Build history of the part. All positions in model axes, mm. Give positions to 0.01 mm unless a question says otherwise; leave off trailing zeros. Loops run counter-clockwise (first coordinate to the right, second up) from the corner with the lowest first, then second, coordinate; pieces in that order, holes last.
1) Band-saw the part on B-B on y = 38.1. List the corners of the cut face in (x, z) (3 decimals).
2) Wall check: line 1 (Y direction, x = 1.25, z = 234) (3 decimals); line 2 (Y direction, x = 5.75, z = -272) (3 decimals); line 3 (Z direction, x = 1, y = 59). Give the ranges that are in metal, low to high.
3) Band-saw the part on A-A on z = -190. List the corners of the cut face in (x, y) (3 decimals).
4) Band-saw the part on C-C on x = 3. List the corners of the cut face in (y, z) (3 decimals), then the cut area to 3 significant figures.
Autodesk Inventor part; units mm, degrees
ref_plane "YZ Plane" through (0, 0, 0) normal (1, 0, 0) x (0, 1, 0)
ref_plane "XZ Plane" through (0, 0, 0) normal (0, 1, 0) x (-1, 0, 0)
ref_plane "XY Plane" through (0, 0, 0) normal (0, 0, 1) x (1, 0, 0)
sketch "Sketch1" plane through (0, 0, 0) normal (1, 0, 0) x (0, 1, 0)
  line L0 (-69.85, 342.9) -> (-69.85, -342.9)
  line L1 (-69.85, -342.9) -> (69.85, -342.9)
  line L2 (69.85, -342.9) -> (69.85, 342.9)
  line L3 (69.85, 342.9) -> (-69.85, 342.9)
  line L4 (-69.85, 342.9) -> (69.85, -342.9) construction
  line L5 (-69.85, -342.9) -> (69.85, 342.9) construction
  point P0 (0, 0)
  dimension "width" = 685.8
  dimension "height" = 139.7
extrude "Extrusion1" add sketch "Sketch1" along normal blind 6.35
sketch "Sketch2" plane through (6.35, 0, 0) normal (1, 0, 0) x (0, 0, -1)
  line L0 (-317.5, 38.1) -> (-63.5, 38.1) construction
  line L1 (-317.5, 28.575) -> (-63.5, 28.575)
  line L2 (-63.5, 47.625) -> (-317.5, 47.625)
  arc A0 (-317.5, 47.625) -> (-317.5, 28.575) centre (-317.5, 38.1) ccw
  arc A1 (-63.5, 28.575) -> (-63.5, 47.625) centre (-63.5, 38.1) ccw
  line L3 (342.9, 69.85) -> (-342.9, 69.85)
  line L4 (-342.9, 69.85) -> (-342.9, -69.85)
  line L5 (63.5, -38.1) -> (317.5, -38.1) construction
  line L6 (63.5, -47.625) -> (317.5, -47.625)
  line L7 (317.5, -28.575) -> (63.5, -28.575)
  arc A2 (63.5, -28.575) -> (63.5, -47.625) centre (63.5, -38.1) ccw
  arc A3 (317.5, -47.625) -> (317.5, -28.575) centre (317.5, -38.1) ccw
  line L8 (-342.9, -69.85) -> (342.9, -69.85)
  line L9 (342.9, -69.85) -> (342.9, 69.85)
  point P0 (0, 0)
  point P1 (-190.5, 38.1)
  point P2 (190.5, -38.1)
  dimension "slot_center_from_top" = 31.75
  dimension "slot_center_from_side" = 152.4
  dimension "slot_radius" = 9.525
  dimension "d7" = 31.75
  dimension "d8" = 152.4
  dimension "d9" = 9.525
  dimension "length_of_slot" = 254
  dimension "d13" = 254
extrude "Extrusion2" cut sketch "Sketch2" against normal through all contours A0 L2 A1 L1 | A2 L7 A3 L6
sketch "Sketch3" plane through (0, 0, 0) normal (-1, 0, 0) x (0, 0, 1)
  line L0 (-342.9, 69.85) -> (342.9, 69.85) construction
  line L1 (6.3584, 69.85) -> (6.3584, -72.7678) construction
  line L2 (342.9, 69.85) -> (342.9, -69.85) construction
  line L3 (-6.3584, 69.85) -> (-6.3584, -69.85) construction
  line L4 (-342.9, -69.85) -> (-342.9, 69.85) construction
  line L5 (-6.3584, 61.976) -> (6.3584, 61.976) construction
  line L6 (-6.3584, -61.976) -> (6.3584, -61.976) construction
  line L7 (342.9, -69.85) -> (-342.9, -69.85) construction
  line L8 (-6.3584, 14.224) -> (6.3584, 14.224) construction
  line L9 (-6.3584, -14.224) -> (6.3584, -14.224) construction
  point P0 (0, 0)
  point P1 (80.6051, 237.827)
  point P2 (47.886, -92.9067)
  dimension "Vertical_Line_For_Bolt_Holes" = 336.5416
  dimension "d15" = 336.5416
  dimension "First_Horizontal_Line" = 7.874
  dimension "d17" = 7.874
  dimension "Second_Horizontal_Line" = 47.752
  dimension "d19" = 47.752
hole "Hole1" at (0, 61.976, 6.3584) at (0, -61.976, -6.3584) at (0, 237.827, 80.6051) at (0, -92.9067, 47.886) at (0, 14.224, 6.3584) at (0, -14.224, -6.3584) direction (1, 0, 0) diameter 6.7564 end through all
equation "\"d9\" = slot_radius"
equation "\"d13\" = length_of_slot"
equation "\"d15\" = Vertical_Line_For_Bolt_Holes"
equation "\"d17\" = First_Horizontal_Line"
properties part number "5.5 x 27 x 1/4/ x 3/8" material "Aluminum 6061"
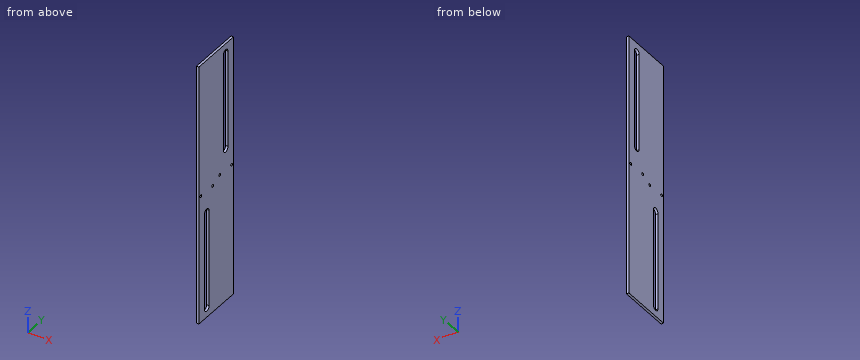
Findings below:
1. outline: (0, -342.9) - (6.35, -342.9) - (6.35, 53.975) - (0, 53.975) - close; (0, 327.025) - (6.35, 327.025) - (6.35, 342.9) - (0, 342.9) - close
2. line 1: y = -69.85 to 28.575, 47.625 to 69.85
2. line 2: y = -69.85 to -47.625, -28.575 to 69.85
2. line 3: z = -342.9 to 4.76, 7.96 to 342.9
3. outline: (0, -69.85) - (6.35, -69.85) - (6.35, -47.625) - (0, -47.625) - close; (0, -28.575) - (6.35, -28.575) - (6.35, 69.85) - (0, 69.85) - close
4. outline: (-69.85, -342.9) - (69.85, -342.9) - (69.85, 342.9) - (-69.85, 342.9) - close; hole circle Ø6.756 at (-61.976, -6.358); hole (-47.625, -317.5) arc R9.525 ccw to (-28.575, -317.5) - (-28.575, -63.5) arc R9.525 ccw to (-47.625, -63.5) - close; hole circle Ø6.756 at (-14.224, -6.358); hole circle Ø6.756 at (14.224, 6.358); hole (28.575, 63.5) arc R9.525 ccw to (47.625, 63.5) - (47.625, 317.5) arc R9.525 ccw to (28.575, 317.5) - close; hole circle Ø6.756 at (61.976, 6.358)
4. area: 85,400 mm2
